Input: part model. Units: mm. Frame: model coordinates. A direction names the side the tool comes from. Give positions to 0.01 mm unless a question says otherwise; leave off trailing zeros. Loops run counter-clockwise (first coordinate to the right, second up) from the corner with the lowest first, then second, coordinate; pieces in that order, holes last. Notation, with made-up numbers: (4.5, 62.25) - (57.5, 62.25) arc R17 cw to (57.5, 70.25) - close; hole circle Ø3 at (-6, 40). An arc over 180 degrees is marked (long way). Answer as a JSON object with one key per item and string values. Group by question number.
(1) Pin query (flat end, axial travel): P1, Ø6, axis at y = 4.5, z = -23, coming from the -X side; P2, Ø6, axis at x = 3.5, y = 2.5, coming from the -Z side; P3, Ø2, axis at x = -3, z = -12.5, coming from the -Y side; P4, Ø5.5, axis at x = 0.5, y = -1, coming from the -Z side. Return the tip coordinate at first contact, or that it passes through.
(2) Section query B-B (y = -0.5). Return loops of the section in (x, z).
(3) Section query A-A (x = 0). Return loops of the section in (y, z).
(4) Material intervals for L1, parallel to X at y = 0, z = -23.25; L2, parallel to Z at x = 1.25, y = -2.5; L3, parallel to Y at x = -2.25, z = -22.5, sorted ascending.
(5) Access query for faces 1 (the flat face through (0.1, -2.5, -15)), 2 (the flat face through (0, 4, -30)). Directions: +Z, -Z, +X, -X, +Y, -Y. A direction counts if a zero-diameter tool reaches every point of the face in a straight line with its end or side. Return the directions, or none.
(6) Section query D-D (y = -3). Return loops of the section in (x, z), plus the area to 3 significant figures.
(7) Section query C-C (z = -6.5). Return loops of the section in (x, y), plus the area to 3 significant figures.
(8) Mould query, pull axis X, two halves, no side actions, for faces 3 (the cylindrical face through (-1.802, 5.723, -15.21)), 4 (the flat face through (0, 1.5, -10)), 5 (the flat face through (0, 3, 0)). Classes: +X half, -X half, draft (parallel to the pull), parting line (faces both ways), or undercut.
```python
from build123d import *
from build123d.topology import SkipClean

# Parameters (mm, degrees)
ESQUISSE1_W             = 30
ESQUISSE1_H             = 6
ENL_V_MAT_EXTRU_4_DEPTH = 5
ENL_V_MAT_EXTRU_5_DEPTH = 18
ENL_V_MAT_EXTRU_6_DEPTH = 15


with BuildPart() as part:
    # Esquisse1 → Révolution1 (revolve)
    with BuildSketch(Plane(origin=(0, 0, 0), x_dir=(0, 0, -1), z_dir=(1, 0, 0)), mode=Mode.PRIVATE) as r_volution1_sk:
        with Locations((15, -3)):
            Rectangle(ESQUISSE1_W, ESQUISSE1_H)
    revolve(r_volution1_sk.sketch.rotate(Axis((0, 0, -30), (0, 0, 1)), 180), axis=Axis((0, 0, -30), (0, 0, 1)))

    # Esquisse2 → Enlèv. mat.-Extru.4 (cut)
    with BuildSketch(Plane.XY):
        with BuildLine():
            Line((-1.677050983, 1.5), (0, 1.5))
            Line((0, 1.5), (1.677050983, 1.5))
            ThreePointArc((1.677050983, 1.5), (0, 2.25), (-1.677050983, 1.5))
        make_face()
    extrude(amount=-ENL_V_MAT_EXTRU_4_DEPTH, mode=Mode.SUBTRACT)

    # Esquisse5 → Enlèv. mat.-Extru.5 (cut)
    with SkipClean():  # the faces are left unmerged after this step: merging them gives an invalid solid
        with BuildSketch(Plane.XY):
            with BuildLine():
                Line((-1.677050983, 1.5), (1.677050983, 1.5))
                ThreePointArc((1.677050983, 1.5), (0, -2.25), (-1.677050983, 1.5))
            make_face()
        extrude(amount=-ENL_V_MAT_EXTRU_5_DEPTH, mode=Mode.SUBTRACT)

    # Esquisse3 → Enlèv. mat.-Extru.6 (cut)
    with BuildSketch(Plane(origin=(0, 0, -30), x_dir=(-1, 0, 0), z_dir=(0, 0, -1))):
        with BuildLine():
            Line((3.620032518, 2.673081474), (-3.620032518, 2.673081474))
            ThreePointArc((-3.620032518, 2.673081474), (-1.407098729, -4.274350613), (4.5, 0))
            ThreePointArc((4.5, 0), (4.274350613, 1.407098729), (3.620032518, 2.673081474))
        make_face()
    extrude(amount=-ENL_V_MAT_EXTRU_6_DEPTH, mode=Mode.SUBTRACT)


solid = part.part
```
Recorded:
{
 "1": {"P1": "stops at x = -5.81", "P2": "stops at z = -30", "P3": "stops at y = -5.66", "P4": "stops at z = -15"},
 "2": {"outline": "(-5.98, -30) - (-4.47, -30) - (-4.47, -15) - (-2.19, -15) - (-2.19, 0) - (-5.98, 0) - close; (2.19, -15) - (4.47, -15) - (4.47, -30) - (5.98, -30) - (5.98, 0) - (2.19, 0) - close"},
 "3": {"outline": "(-6, -30) - (-4.5, -30) - (-4.5, -15) - (-2.25, -15) - (-2.25, 0) - (-6, 0) - close; (1.5, -15) - (2.67, -15) - (2.67, -30) - (6, -30) - (6, 0) - (2.25, 0) - (2.25, -5) - (1.5, -5) - close"},
 "4": {"L1": "x = -6 to -4.5, 4.5 to 6", "L2": "z = -15 to 0", "L3": "y = -5.56 to -3.9, 2.67 to 5.56"},
 "5": {"face 1": "-Z", "face 2": "-Z, +X, -X, +Y, -Y"},
 "6": {"outline": "(-5.2, -30) - (-3.35, -30) - (-3.35, -15) - (3.35, -15) - (3.35, -30) - (5.2, -30) - (5.2, 0) - (-5.2, 0) - close", "area": "211 mm^2"},
 "7": {"outline": "circle Ø12 at (0, 0); hole (-1.68, 1.5) arc R2.25 ccw (long way) to (1.68, 1.5) - close", "area": "98.9 mm^2"},
 "8": {"face 3": "parting line", "face 4": "undercut", "face 5": "draft"}
}
